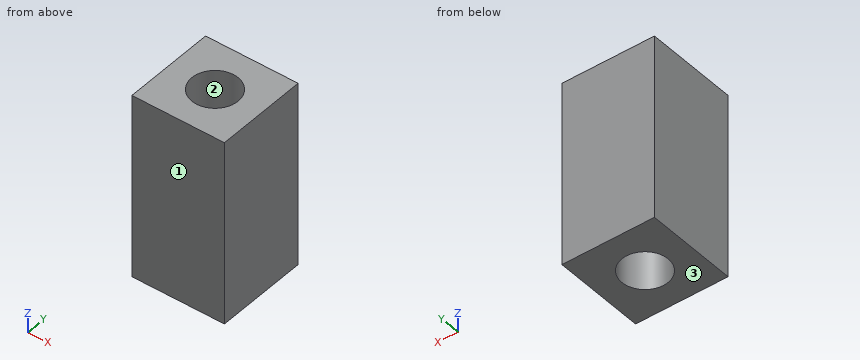
Autodesk Inventor part; units mm, degrees
ref_plane "YZ Plane" through (0, 0, 0) normal (1, 0, 0) x (0, 1, 0)
ref_plane "XZ Plane" through (0, 0, 0) normal (0, 1, 0) x (-1, 0, 0)
ref_plane "XY Plane" through (0, 0, 0) normal (0, 0, 1) x (1, 0, 0)
sketch "Sketch1" plane through (0, 0, 0) normal (0, 0, 1) x (1, 0, 0)
  line L0 (0, 0) -> (12.7, 0)
  line L1 (12.7, 0) -> (12.7, -12.7)
  line L2 (12.7, -12.7) -> (0, -12.7)
  line L3 (0, -12.7) -> (0, 0)
  circle A0 centre (6.35, -6.35) radius 3.175
  dimension "d0" = 6.35
  dimension "d1" = 12.7
  dimension "d2" = 12.7
  dimension "d3" = 6.35
  dimension "d4" = 6.35
extrude "Extrusion1" add sketch "Sketch1" along normal blind 25.4
properties part number "boltholder" material "Aluminum 6061"
CAD build for the part. Positions are in the model's coordinates, mm. Face numbers are marked on the shaded views. Round coordinates to 2 decimals unless told otherwise and drop trailing zeros. Order: outer loops, then holes, each group sorted by start corner. A loop starts at its lowest first (then second) coordinate and runs counter-clockwise, first axis right, second up.
Q1. Wall check: L1, parallel to Y at x = 6.35, z = 15 (3 decimals); L2, parallel to Y at x = 3.5, z = 22.5; L3, parallel to X at y = -9.25, z = 21. Give the ranges that are in metal, low to high.
Q2. Slice it at A-A (y = -6.35). Write the cut outline in (x, z) (3 decimals).
Q3. Two-plate mould, pull along Y, no slides. Class the marked faces 1, 2 and 3: pulls with the +Y half, pulls with the -Y half, needs draft (parallel to the pull), parting line crosses it, or undercut.
Q4. Slice it at C-C (z = 7). Write the cut outline in (x, y) (3 decimals), and give its area (3 significant figures).
Q5. Slice it at B-B (x = 6.35). Write the cut outline in (y, z) (3 decimals), and give its area (3 significant figures).
Results below:
1. L1: y = -12.7 to -9.525, -3.175 to 0
1. L2: y = -12.7 to -7.75, -4.95 to 0
1. L3: x = 0 to 5.06, 7.64 to 12.7
2. outline: (0, 0) - (3.175, 0) - (3.175, 25.4) - (0, 25.4) - close; (9.525, 0) - (12.7, 0) - (12.7, 25.4) - (9.525, 25.4) - close
3. face 1: pulls with the -Y half
3. face 2: undercut
3. face 3: needs draft
4. outline: (0, -12.7) - (12.7, -12.7) - (12.7, 0) - (0, 0) - close; hole circle Ø6.35 at (6.35, -6.35)
4. area: 130 mm2
5. outline: (-12.7, 0) - (-9.525, 0) - (-9.525, 25.4) - (-12.7, 25.4) - close; (-3.175, 0) - (0, 0) - (0, 25.4) - (-3.175, 25.4) - close
5. area: 161 mm2
